Read the model definition and answer for the solid it produces. Units are mm, in the model's axes. Face numbers are marked on the shaded views. Give positions to 0.01 mm unless a question says otherwise; leave off trailing zeros. Order: outer loops, then holes, each group sorted by start corner. A loop starts at its lowest first (then second) coordinate and runs counter-clockwise, first axis right, second up. Notation, with made-up numbers: (82, 27) -> (115, 27) arc R12 ccw to (115, 34) -> close; hole circle Ø2 at (63, 44.25). An arc over 180 degrees is marked (long way). Answer as CSV lines item,"result". Start each with the question number.
1) Find section C-C (z = -30). Determine the outline of the cut face in (x, y), and give its area (3 significant figures).
2) Find section D-D (x = 1.1). Determine the outline of the cut face in (y, z).
3) Find section A-A (x = 4.3). Determine the outline of the cut face in (y, z).
4) Flat-ended cylindrical pins translate along their axes: pin 1 Ø2 at (y, z) = (2, 0) entering from +X; pin 2 Ø2 at (x, y) = (4.5, 0.5) entering from +Z; pin 3 Ø1.5 at (x, y) = (4.5, 14) entering from +Z. Find the tip coordinate at first contact, or state that the pin passes through.
5) The mould has two halves that part along Y. Classify the marked faces 1, 2 and 3: +Y half, -Y half, draft (parallel to the pull), parting line (faces both ways), or undercut.
6) Find section B-B (y = 0). Determine the outline of the cut face in (x, z), and give its area (3 significant figures).
7) Straight lines are drawn through the part: L1, parallel to Y at x = 3.2, z = -19.5; L2, parallel to X at y = -13.5, z = -18; L3, parallel to Z at x = 4.4, y = 1. For each, find the intervals that lie inside material, in ascending order. Write a range as from..to.
```python
from build123d import *

# Parameters (mm, degrees)
BOSS_EXTRUDE1_DEPTH = 5
SHELL1_T            = -3


with BuildPart() as part:
    # Sketch1 → Boss-Extrude1 (new body)
    with BuildSketch(Plane(origin=(0, 0, 0), x_dir=(0, 0, -1), z_dir=(1, 0, 0))):
        with BuildLine():
            Line((0, 18), (45, 18))
            Line((45, 18), (45, -18))
            Line((45, -18), (0, -18))
            ThreePointArc((0, -18), (-18, 0), (0, 18))
        make_face()
    extrude(amount=BOSS_EXTRUDE1_DEPTH)

    # Shell1
    shell1_openings = [part.faces().sort_by_distance(p)[0] for p in [
        (5, 0, -15.294949805),
    ]]
    offset(amount=SHELL1_T, openings=shell1_openings, kind=Kind.INTERSECTION)


solid = part.part
```
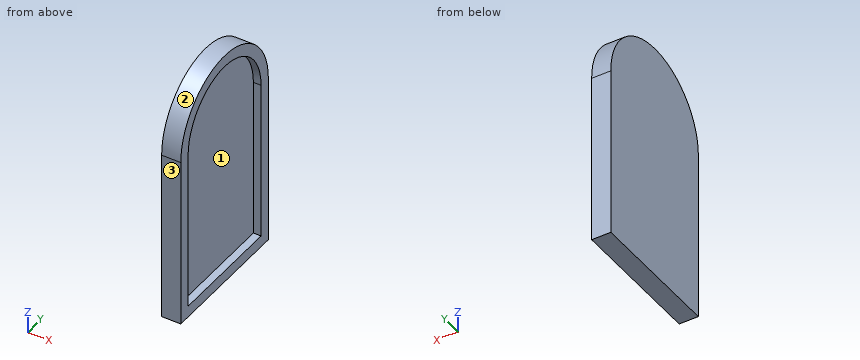
Findings below:
1,outline,"(0, -18) -> (5, -18) -> (5, -15) -> (3, -15) -> (3, 15) -> (5, 15) -> (5, 18) -> (0, 18) -> close"
1,area,"120 mm²"
2,outline,"(-18, -45) -> (18, -45) -> (18, 0) arc R18 ccw to (-18, 0) -> close"
3,outline,"(-18, -45) -> (18, -45) -> (18, 0) arc R18 ccw to (-18, 0) -> close; hole (-15, -42) -> (15, -42) -> (15, 0) arc R15 ccw to (-15, 0) -> close"
4,pin 1,"x = 3"
4,pin 2,"z = 18"
4,pin 3,"z = 12.18"
5,face 1,"undercut"
5,face 2,"parting line"
5,face 3,"-Y half"
6,outline,"(0, -45) -> (5, -45) -> (5, -42) -> (3, -42) -> (3, 15) -> (5, 15) -> (5, 18) -> (0, 18) -> close"
6,area,"201 mm²"
7,L1,"-18..-15, 15..18"
7,L2,"0..3"
7,L3,"-45..-42, 14.97..17.97"
